Design review of the part built by this model. Coordinates are the model's own, in mm. Face numbers are marked on the shaded views. A direction names the side the tool comes from. Round coordinates to 2 decimals unless told otherwise and drop trailing zeros. Loops run counter-clockwise (first coordinate to the right, second up) from the corner with the lowest first, then second, coordinate; pieces in that order, holes last. Notation, with made-up numbers: (-35, -31.75) - (-19, -31.75) arc R26 ccw to (-19, -2.75) - close; hole circle Ø1 at (-20, 77.25). An arc over 180 degrees is marked (long way). Answer as CSV lines item,"result". Start each with the question number.
(1) Consider section C-C (y = 4.5). Give the boundary of the cut face in (x, z), and give its area (3 significant figures).
(2) Mouldability with a two-part tool opening along Y and no side actions: class the marked faces 4 and 5 as released by +Y, released by -Y, zero draft, split by the parting line, or undercut.
(3) For the marked faces 1, 2 and 3, list the 3-axis set-ups (+Z, -Z, +X, -X, +Y, -Y) from which the entire face can be reached by the end or side of a thin tool; tool diameter is ignored.
(4) Wall thickness on L1, parallel to X at y = -3, z = -4.5; L2, parallel to X at y = 2.5, z = -4; L3, parallel to Z at x = 69, y = 4.5: over which ranges is each line inside the solid? List them lowest first.
(5) For P1, Ø1, axis at y = 3, z = -4.5, coming from the -X side; P2, Ø4, axis at x = 31.5, y = 4, coming from the -Z side; P3, Ø1.3, axis at x = 44, y = 3, coming from the +Z side; P4, Ø2, axis at x = 33.5, y = -2.5, coming from the -Z side, all flat-tipped, find the tip position at first contact; note any pin that passes through.
(6) Consider section B-B (z = -4.75). Give the boundary of the cut face in (x, y).
(7) Consider section D-D (x = 66.5). Give the boundary of the cut face in (y, z), and give its area (3 significant figures).
(8) Consider section A-A (y = -2.75). Give the boundary of the cut face in (x, z).
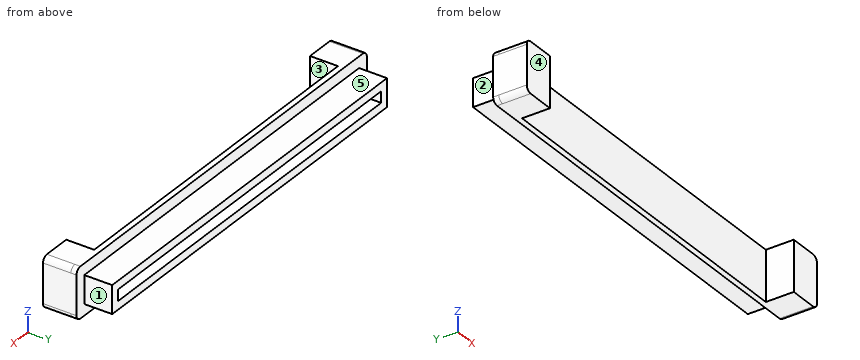
from build123d import *

# Parameters (mm, degrees)
SKETCH1_W           = 75
SKETCH1_H           = 9
BOSS_EXTRUDE1_DEPTH = 1
FILLET1_R           = 1
SKETCH8_W           = 71
SKETCH8_H           = 5
BOSS_EXTRUDE2_DEPTH = 6
SHELL1_T            = -1.5
SKETCH9_W           = 6
SKETCH9_H           = 9
BOSS_EXTRUDE3_DEPTH = 5
LPATTERN1_COUNT     = 2
LPATTERN1_PITCH     = 69
FILLET2_R           = 1


with BuildPart() as part:
    # Sketch1 → Boss-Extrude1 (new body)
    with BuildSketch(Plane(origin=(0, 0, 0), x_dir=(1, 0, 0), z_dir=(0, 1, 0))):
        with Locations((37.5, 4.5)):
            Rectangle(SKETCH1_W, SKETCH1_H)
    extrude(amount=BOSS_EXTRUDE1_DEPTH)

    # Fillet1
    fillet1_edges = [part.edges().sort_by_distance(p)[0] for p in [
        (0, 0.5, -9),
        (75, 0.5, -9),
        (75, 0.5, 0),
        (0, 0.5, 0),
    ]]
    fillet(fillet1_edges, radius=FILLET1_R)

    # Sketch8 → Boss-Extrude2 (add)
    with BuildSketch(Plane(origin=(0, 0, 0), x_dir=(1, 0, 0), z_dir=(0, 1, 0))):
        with Locations((37.5, 4.5)):
            Rectangle(SKETCH8_W, SKETCH8_H)
    extrude(amount=BOSS_EXTRUDE2_DEPTH)

    # Shell1
    shell1_openings = [part.faces().sort_by_distance(p)[0] for p in [
        (37.5, 6, -4.5),
    ]]
    offset(amount=SHELL1_T, openings=shell1_openings, kind=Kind.INTERSECTION)

    # Sketch9 → Boss-Extrude3 (add)
    with BuildSketch(Plane(origin=(0, 0, 0), x_dir=(-1, 0, 0), z_dir=(0, -1, 0))):
        with Locations((-3, 4.5)):
            Rectangle(SKETCH9_W, SKETCH9_H)
    boss_extrude3 = extrude(amount=BOSS_EXTRUDE3_DEPTH)

    # LPattern1: Boss-Extrude3 ×2
    with Locations(*[(i * LPATTERN1_PITCH, 0, 0) for i in range(1, LPATTERN1_COUNT)]):
        add(boss_extrude3)

    # Fillet2
    fillet2_edges = [part.edges().sort_by_distance(p)[0] for p in [
        (0, -2.5, 0),
        (0, -2.5, -9),
        (75, -2.5, -9),
        (75, -2.5, 0),
    ]]
    fillet(fillet2_edges, radius=FILLET2_R)


solid = part.part
Determined:
1,outline,"(2, -7) - (73, -7) - (73, -2) - (2, -2) - close; hole (3.5, -5.5) - (71.5, -5.5) - (71.5, -3.5) - (3.5, -3.5) - close"
1,area,"219 mm^2"
2,face 4,"released by -Y"
2,face 5,"zero draft"
3,face 1,"+Z, -Z, +X, +Y"
3,face 2,"+Z, -Z, -X, +Y"
3,face 3,"+Z, -Z, -Y"
4,L1,"x = 0 to 6, 69 to 75"
4,L2,"x = 2 to 3.5, 71.5 to 73"
4,L3,"z = -7 to -5.5, -3.5 to -2"
5,P1,"stops at x = 2"
5,P2,"stops at z = -7"
5,P3,"stops at z = -2"
5,P4,"passes through"
6,outline,"(0, -5) - (6, -5) - (6, 0) - (69, 0) - (69, -5) - (75, -5) - (75, 1) - (73, 1) - (73, 6) - (71.5, 6) - (71.5, 1.5) - (3.5, 1.5) - (3.5, 6) - (2, 6) - (2, 1) - (0, 1) - close"
7,outline,"(0, -9) - (1, -9) - (1, -7) - (6, -7) - (6, -5.5) - (1.5, -5.5) - (1.5, -3.5) - (6, -3.5) - (6, -2) - (1, -2) - (1, 0) - (0, 0) - close"
7,area,"25.0 mm^2"
8,outline,"(0, -8) arc R1 ccw to (1, -9) - (6, -9) - (6, 0) - (1, 0) arc R1 ccw to (0, -1) - close; (69, -9) - (74, -9) arc R1 ccw to (75, -8) - (75, -1) arc R1 ccw to (74, 0) - (69, 0) - close"
